Model file for the job. Use its own axes, mm. Face numbers are marked on the shaded views. Give positions to 0.01 mm unless a question says otherwise; leave off trailing zeros. Write each loop counter-clockwise with the first axis right and the second up, starting at its lowest first coordinate (ties: lowest second). Pieces come first, ordered by that corner, then holes. Notation, with made-up numbers: (85, -23.5) - (121, -23.5) arc R27 cw to (121, 1.5) - close; hole circle Ø1 at (83.25, 22.25). An arc over 180 degrees is marked (long way). One line per item, written item: value. Start each with the question number.
(1) Probe L1, parallel to X at y = 0.25, z = 25; L2, parallel to Z at x = 12.5, y = -7; L3, parallel to X at y = 10.75, z = 22.5. List the from-to ranges inside material, lowest first.
(2) Cut at D-D, the plane y = -6.5. List the corners of the cut face in (x, z).
(3) Cut at C-C, the plane x = 15. List the corners of the cut face in (y, z).
(4) Cut at A-A, the plane y = 0. List the corners of the cut face in (x, z), and give its area (3 significant figures).
(5) Cut at B-B, the plane z = 25. List the corners of the cut face in (x, y).
(6) Drop a flat-ended pin along its axis: P1, Ø1.5, axis at x = 8, z = -3, coming from the +Y side. Give the stop position or say it passes through.
(7) Mould opens along X. For the marked faces 1, 2, 3 and 4 say: pulls with the +X half, pulls with the -X half, needs draft (parallel to the pull), parting line crosses it, or undercut.
Autodesk Inventor part; units mm, degrees
ref_plane "YZ Plane" through (0, 0, 0) normal (1, 0, 0) x (0, 1, 0)
ref_plane "XZ Plane" through (0, 0, 0) normal (0, 1, 0) x (-1, 0, 0)
ref_plane "XY Plane" through (0, 0, 0) normal (0, 0, 1) x (1, 0, 0)
sketch "Sketch1" plane through (0, 0, 0) normal (0, 0, 1) x (1, 0, 0)
  line L0 (-17.5, -12.5) -> (17.5, -12.5)
  line L1 (17.5, -12.5) -> (17.5, 12.5)
  line L2 (17.5, 12.5) -> (-17.5, 12.5)
  line L3 (-17.5, 12.5) -> (-17.5, -12.5)
  line L4 (-17.5, -12.5) -> (17.5, 12.5) construction
  line L5 (17.5, -12.5) -> (-17.5, 12.5) construction
  point P0 (0, 0)
  dimension "d0" = 35
  dimension "d1" = 25
extrude "Extrusion1" add sketch "Sketch1" along normal blind 30
sketch "Sketch2" plane through (0, 0, 0) normal (0, 0, -1) x (-1, 0, 0)
  circle A0 centre (0, 0) radius 12.5
  dimension "d4" = 25
extrude "Extrusion2" add sketch "Sketch2" along normal blind 10
sketch "Sketch3" plane through (-17.5, 12.5, 30) normal (0, 1, 0) x (1, 0, 0)
  circle A0 centre (30, 5) radius 3.5
  circle A1 centre (5, 5) radius 3.5
  line L0 (35, 0) -> (0, 0)
  line L1 (0, 30) -> (0, 0)
  line L2 (35, 30) -> (35, 0)
  point P0 (17.5, 30)
  dimension "d7" = 7
  dimension "d8" = 7
  dimension "d9" = 5
  dimension "d10" = 5
  dimension "d11" = 5
  dimension "d12" = 5
extrude "Extrusion3" cut sketch "Sketch3" against normal through all
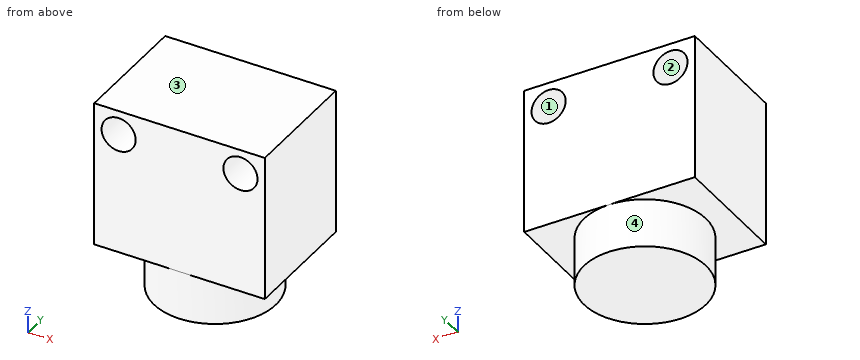
Answers follow:
1. L1: x = -17.5 to -16, -9 to 9, 16 to 17.5
1. L2: z = 0 to 21.5, 28.5 to 30
1. L3: x = -17.5 to -14.95, -10.05 to 10.05, 14.95 to 17.5
2. outline: (-17.5, 0) - (-10.68, 0) - (-10.68, -10) - (10.68, -10) - (10.68, 0) - (17.5, 0) - (17.5, 30) - (-17.5, 30) - close; hole circle Ø7 at (-12.5, 25); hole circle Ø7 at (12.5, 25)
3. outline: (-12.5, 0) - (12.5, 0) - (12.5, 22.55) - (-12.5, 22.55) - close; (-12.5, 27.45) - (12.5, 27.45) - (12.5, 30) - (-12.5, 30) - close
4. outline: (-17.5, 0) - (-12.5, 0) - (-12.5, -10) - (12.5, -10) - (12.5, 0) - (17.5, 0) - (17.5, 30) - (-17.5, 30) - close; hole circle Ø7 at (-12.5, 25); hole circle Ø7 at (12.5, 25)
4. area: 1,220 mm²
5. outline: (-17.5, -12.5) - (-16, -12.5) - (-16, 12.5) - (-17.5, 12.5) - close; (-9, -12.5) - (9, -12.5) - (9, 12.5) - (-9, 12.5) - close; (16, -12.5) - (17.5, -12.5) - (17.5, 12.5) - (16, 12.5) - close
6. P1: stops at y = 10.18
7. face 1: undercut
7. face 2: undercut
7. face 3: needs draft
7. face 4: parting line crosses it
